Can you work these out from the model? Positions are in its coordinate system, mm. A direction names the side the tool comes from. Round coordinates to 2 decimals unless told otherwise and drop trailing zeros. Loops run counter-clockwise (first coordinate to the right, second up) from the corner with the lowest first, then second, coordinate; pieces in that order, holes last. Notation, with made-up numbers: (-23.5, 79) -> (-18.5, 79) arc R34 ccw to (-18.5, 110) -> close; hole circle Ø1 at (42, 11). An arc over 180 degrees is marked (long way). Use a Markdown table: item, result.
from build123d import *

# Parameters (mm, degrees)
BOSS_EXTRUDE1_DEPTH       = 1.6002
F_0_CLEARANCE_HOLE1_D     = 1.778
F_0_CLEARANCE_HOLE1_DEPTH = 465
F_0_CLEARANCE_HOLE1_TIP   = 0.53416509
F_0_CLEARANCE_HOLE2_D     = 1.778
F_0_CLEARANCE_HOLE2_DEPTH = 465
F_0_CLEARANCE_HOLE2_TIP   = 0.53416509


with BuildPart() as part:
    # Sketch1 → Boss-Extrude1 (new body)
    with BuildSketch(Plane.XY):
        with BuildLine():
            Line((1.827005239, -2.620493359), (18.4125, -2.620493359))
            ThreePointArc((18.4125, -2.620493359), (19.535032015, -2.155525374), (20, -1.032993359))
            Line((20, -1.032993359), (20, 0.792006641))
            ThreePointArc((20, 0.792006641), (19.535032015, 1.914538656), (18.4125, 2.379506641))
            Line((18.4125, 2.379506641), (1.827005239, 2.379506641))
            ThreePointArc((1.827005239, 2.379506641), (-2.977484791, 0.366857357), (1.194771818, -2.75182127))
            ThreePointArc((1.194771818, -2.75182127), (1.504140671, -2.653672053), (1.827005239, -2.620493359))
        make_face()
    extrude(amount=BOSS_EXTRUDE1_DEPTH)

    # #0 Clearance Hole1
    with Locations(Plane.XY.offset(1.6002)):
        with Locations((0, 0)):
            Hole(F_0_CLEARANCE_HOLE1_D / 2, depth=F_0_CLEARANCE_HOLE1_DEPTH)
            with Locations((0, 0, -(F_0_CLEARANCE_HOLE1_DEPTH + F_0_CLEARANCE_HOLE1_TIP / 2))):  # 118° drill point
                Cone(0, F_0_CLEARANCE_HOLE1_D / 2, F_0_CLEARANCE_HOLE1_TIP, mode=Mode.SUBTRACT)

    # #0 Clearance Hole2
    with Locations(Plane(origin=(0, 0, 0), x_dir=(-1, 0, 0), z_dir=(0, 0, -1))):
        with Locations((-16.993218834, 0.022656086)):
            Hole(F_0_CLEARANCE_HOLE2_D / 2, depth=F_0_CLEARANCE_HOLE2_DEPTH)
            with Locations((0, 0, -(F_0_CLEARANCE_HOLE2_DEPTH + F_0_CLEARANCE_HOLE2_TIP / 2))):  # 118° drill point
                Cone(0, F_0_CLEARANCE_HOLE2_D / 2, F_0_CLEARANCE_HOLE2_TIP, mode=Mode.SUBTRACT)


solid = part.part
1. I want a section at D-D (y = -1.6). Please give me the cut outline in (x, z).
Answer sheet:
| item | result |
|---|---|
| outline | (-2.54, 0) -> (19.9, 0) -> (19.9, 1.6) -> (-2.54, 1.6) -> close |
2. Will these pins go through, and if not, where does the flat tip stop? pin 1 Ø0.8 at (x, z) = (7, 1) entering from +Y; pin 2 Ø0.5 at (x, z) = (11, 0.5) entering from -Y; pin 3 Ø1.6 at (x, y) = (0, 0) entering from +Z.
Answer sheet:
| item | result |
|---|---|
| pin 1 | stops at y = 2.38 |
| pin 2 | stops at y = -2.62 |
| pin 3 | passes through |
3. If we mould it in two halves opening along Y, with no side actions, what happens to faces 1 (the flat face through (20, 0, 1)), 2 (the flat face through (10, 2.38, 1)), 3 (the cylindrical face through (0.19, -0.87, 0.79))? For each: +Y half, -Y half, draft (parallel to the pull), parting line (faces both ways), or undercut.
Answer sheet:
| item | result |
|---|---|
| face 1 | draft |
| face 2 | +Y half |
| face 3 | undercut |
4. I want a section at C-C (x = 12.25). Please give me the cut outline in (y, z).
Answer sheet:
| item | result |
|---|---|
| outline | (-2.62, 0) -> (2.38, 0) -> (2.38, 1.6) -> (-2.62, 1.6) -> close |
5. I need wall thicknesses on line 1 (Y direction, x = 0, z = 1.05); line 2 (X direction, y = 0.75, z = 0.15); line 3 (Y direction, x = 9.75, z = 1.5). Which ranges of each line are inside material? Lowest first, please.
Answer sheet:
| item | result |
|---|---|
| line 1 | y = -3 to -0.89, 0.89 to 3 |
| line 2 | x = -2.9 to -0.48, 0.48 to 16.48, 17.5 to 20 |
| line 3 | y = -2.62 to 2.38 |
6. I want a section at B-B (z = 0.3). Please give me the cut outline in (x, y) (1 decimal), plus the area to 3 significant figures.
Answer sheet:
| item | result |
|---|---|
| outline | (1.2, -2.8) arc R1.6 cw to (1.8, -2.6) -> (18.4, -2.6) arc R1.6 ccw to (20, -1) -> (20, 0.8) arc R1.6 ccw to (18.4, 2.4) -> (1.8, 2.4) arc R3 ccw (long way) to start; hole circle Ø1.8 at (0, 0); hole circle Ø1.8 at (17, 0) |
| area | 109 mm² |
7. I want a section at A-A (x = 0). Please give me the cut outline in (y, z).
Answer sheet:
| item | result |
|---|---|
| outline | (-3, 0) -> (-0.89, 0) -> (-0.89, 1.6) -> (-3, 1.6) -> close; (0.89, 0) -> (3, 0) -> (3, 1.6) -> (0.89, 1.6) -> close |
8. Which directions (+Z, -Z, +X, -X, +Y, -Y) give clear straight access to the entire face, cutting with the end or side of a thin tool? Please do faces 4 (the cylindrical face through (19.55, 1.9, 0.79)), 5 (the flat face through (10, -2.62, 1)).
Answer sheet:
| item | result |
|---|---|
| face 4 | +Z, -Z, +X, +Y |
| face 5 | +Z, -Z, +X, -Y |
